Check sheet for the modelled part. Datum: model origin and axes. Units: mm. A direction names the side the tool comes from. Give positions to 0.01 mm unless a question says otherwise; leave off trailing zeros. Order: outer loops, then holes, each group sorted by start corner. A loop starts at its lowest first (then second) coordinate and runs counter-clockwise, first axis right, second up.
Autodesk Inventor part; units mm, degrees
ref_plane "Work Plane1" through (-30.4, 7.5, 0) normal (1, 0, 0) x (0, 0, -1)
ref_plane "YZ Plane" through (0, 0, 0) normal (1, 0, 0) x (0, 1, 0)
ref_plane "XZ Plane" through (0, 0, 0) normal (0, 1, 0) x (-1, 0, 0)
sketch "Sketch1" plane through (0, 0, 0) normal (0, 0, 1) x (1, 0, 0)
  line L0 (0, 0) -> (0, 15)
  line L1 (0, 15) -> (5, 15)
  line L2 (5, 15) -> (5, 7.5)
  line L3 (5, 7.5) -> (10.2, 7.5)
  line L4 (10.2, 7.5) -> (10.2, 15)
  line L5 (10.2, 15) -> (15.2, 15)
  line L6 (15.2, 15) -> (15.2, 0)
  line L7 (15.2, 0) -> (0, 0)
  dimension "d0" = 15
  dimension "d1" = 5.2
  dimension "d2" = 5
  dimension "d3" = 5
  dimension "d4" = 7.5
extrude "Extrusion1" add sketch "Sketch1" along normal blind 5
mirror "Mirror1" about plane through (15.2, 0, 0) normal (1, 0, 0) of "Extrusion1"
mirror "Mirror2" about plane through (30.4, 15, 0) normal (1, 0, 0) of "Extrusion1", "Mirror1"
mirror "Mirror3" about plane through (60.8, 15, 0) normal (1, 0, 0) of "Extrusion1", "Mirror1", "Mirror2"
mirror "Mirror4" about plane through (0, 15, 0) normal (-1, 0, 0) of "Extrusion1"
mirror "Mirror5" about plane through (-15.2, 0, 0) normal (-1, 0, 0) of "Extrusion1", "Mirror4"
ref_plane "Work Plane1" through (-30.4, 7.5, 0) normal (1, 0, 0) x (0, 0, -1)
mirror "Mirror6" about plane through (-30.4, 7.5, 0) normal (1, 0, 0) of "Extrusion1", "Mirror4"
ref_plane "Work Plane2" through (-30.4, 7.5, 0) normal (1, 0, 0) x (0, 0, -1)
properties part number "brace"
Q1. Go/stop test with a flat-tipped pin: P1, Ø1.5, axis at x = -53.5, z = 1.5, coming from the +Y side. Record where the tip stops, or that it passes through.
Q2. Sectioned sample at A-A, the plane y = 11. Count the separate pieces of the cut face and the enclosed holes in it, plus the area to 3 significant figures.
Q3. Draft check along X on faces 1 (the flat face through (50.6, 11, 2)), 2 (the flat face through (-61, 15, 2)). Enter one of: pulls with the +X half, pulls with the -X half, needs draft (parallel to the pull), parting line crosses it, or undercut.
Q4. Material ranges on line 1 (Y direction, x = -40, z = 0.4), recorded low to high.
Q5. Tool access check on faces 3 (the flat face through (76, 15, 2)), 4 (the flat face through (65.8, 11, 2)). Record the directions out of +Z, -Z, +X, -X, +Y, -Y that give a thin tool (end or side, any length) a straight path to the whole face; none if there is none.
Q6. Sectioned sample at B-B, the plane x = -22. Record the cut outline in (y, z), plus the area to 3 significant figures.
Filled in:
1. P1: stops at y = 7.5
2. separate pieces: 14
2. enclosed holes: 0
2. area: 650 mm2
3. face 1: undercut
3. face 2: needs draft
4. line 1: y = 0 to 7.5
5. face 3: +Z, -Z, +X, -X, +Y
5. face 4: +Z, -Z, +Y
6. outline: (0, 0) - (7.5, 0) - (7.5, 5) - (0, 5) - close
6. area: 37.5 mm2
